Check sheet for the drawn part. Datum: minimum x, y, z corner. Units: mm. A direction names the side the tool comes from. Round coordinates to 2 decimals unless told otherwise and drop trailing zeros. Loops run counter-clockwise (first coordinate to the right, second up) from the corner with the lowest first, then second, coordinate; pieces in that order, holes last. Notation, with made-up numbers: (19, 9) -> (67, 9) arc R14 cw to (67, 21) -> close; hole circle Ø5 at (71.5, 34.5). An arc over 180 degrees is marked (long way). Use CSV: the item, a comma, the result in double quotes. Start each with the question number.
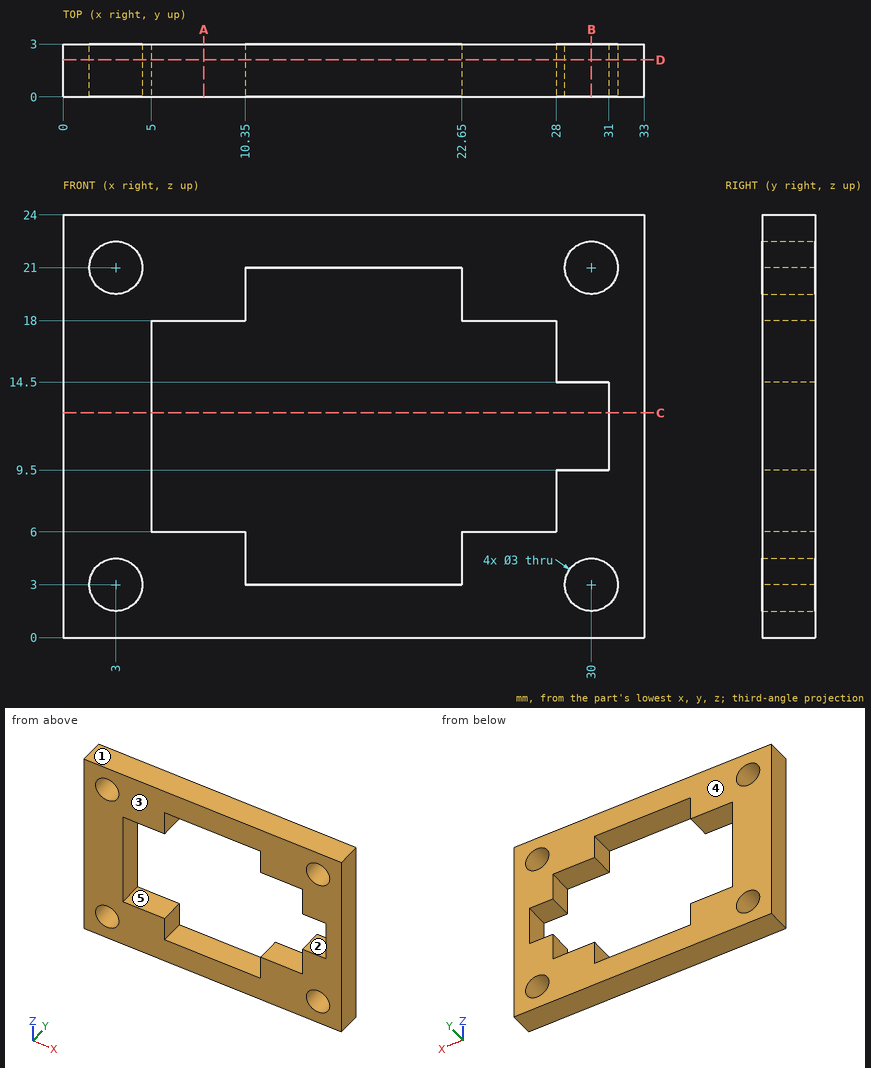
Q1. Release check for a two-part mould opening along Z. For the marked faces 1, 2 and 3 record: +Z half, -Z half, draft (parallel to the pull), parting line (faces both ways), or undercut.
Q2. Cross-section at D-D (y = 2.1). Record the boundary of the cut face in (x, z), and give its area (3 significant figures).
Q3. Depth check by flat-ended pin: pin 1 Ø0.9 at (x, y) = (29.5, 1) entering from -Z. Enter the tip coordinate at first touch or a pass-through.
Q4. Cross-section at A-A (x = 8). Record the boundary of the cut face in (y, z), and give its area (3 significant figures).
Q5. Thickness scan on L1, parallel to Z at x = 3, y = 2.1; L2, parallel to Z at x = 11, y = 1.5; L3, parallel to X at y = 1.75, z = 11. Record the ranges inside material, lowest first. Write a range as from..to.
Q6. Cross-section at C-C (z = 12.75). Record the boundary of the cut face in (x, y).
Q7. Cross-section at B-B (x = 30). Record the boundary of the cut face in (y, z).
Q8. Tool access check on the marked faces 4 and 5. Record the directions out of +Z, -Z, +X, -X, +Y, -Y that give a thin tool (end or side, any length) a straight path to the whole face; none if there is none.
Answer list:
1,face 1,"+Z half"
1,face 2,"undercut"
1,face 3,"draft"
2,outline,"(0, 0) -> (33, 0) -> (33, 24) -> (0, 24) -> close; hole circle Ø3 at (3, 3); hole circle Ø3 at (3, 21); hole (5, 6) -> (10.35, 6) -> (10.35, 3) -> (22.65, 3) -> (22.65, 6) -> (28, 6) -> (28, 9.5) -> (31, 9.5) -> (31, 14.5) -> (28, 14.5) -> (28, 18) -> (22.65, 18) -> (22.65, 21) -> (10.35, 21) -> (10.35, 18) -> (5, 18) -> close; hole circle Ø3 at (30, 3); hole circle Ø3 at (30, 21)"
2,area,"399 mm2"
3,pin 1,"stops at z = 0"
4,outline,"(0, 0) -> (3, 0) -> (3, 6) -> (0, 6) -> close; (0, 18) -> (3, 18) -> (3, 24) -> (0, 24) -> close"
4,area,"36.0 mm2"
5,L1,"z = 0..1.5, 4.5..19.5, 22.5..24"
5,L2,"z = 0..3, 21..24"
5,L3,"x = 0..5, 31..33"
6,outline,"(0, 0) -> (5, 0) -> (5, 3) -> (0, 3) -> close; (31, 0) -> (33, 0) -> (33, 3) -> (31, 3) -> close"
7,outline,"(0, 0) -> (3, 0) -> (3, 1.5) -> (0, 1.5) -> close; (0, 4.5) -> (3, 4.5) -> (3, 9.5) -> (0, 9.5) -> close; (0, 14.5) -> (3, 14.5) -> (3, 19.5) -> (0, 19.5) -> close; (0, 22.5) -> (3, 22.5) -> (3, 24) -> (0, 24) -> close"
8,face 4,"+Z, -Z, +X, -X, +Y"
8,face 5,"+Y, -Y"
